from build123d import *

# Parameters (mm, degrees)
SKETCH1_R           = 2
BOSS_EXTRUDE1_DEPTH = 2.5
FILLET1_R           = 4
FILLET3_R           = 12


with BuildPart() as part:
    # Sketch1 → Boss-Extrude1 (new body)
    with BuildSketch(Plane(origin=(0, 0, 0), x_dir=(1, 0, 0), z_dir=(0, 1, 0))):
        Polygon((-14.798836476, 8.869056619), (-26.798836476, 8.869056619), (-26.798836476, -35.130943381), (199.665714924, -35.130943381), (199.665714924, 8.869056619), (187.665714924, 8.869056619), (187.665714924, -23.130943381), (-14.798836476, -23.130943381), align=None)
        with Locations(Location((-20.798836476, 2.869056619, 0), (0, 0, 270))):
            Circle(SKETCH1_R, mode=Mode.SUBTRACT)
        with Locations(Location((-20.798836476, -29.130943381, 0), (0, 0, 270))):
            Circle(SKETCH1_R, mode=Mode.SUBTRACT)
        with Locations(Location((193.665714924, 2.869056619, 0), (0, 0, 270))):
            Circle(SKETCH1_R, mode=Mode.SUBTRACT)
        with Locations(Location((193.665714924, -29.130943381, 0), (0, 0, 270))):
            Circle(SKETCH1_R, mode=Mode.SUBTRACT)
    extrude(amount=BOSS_EXTRUDE1_DEPTH)

    # Fillet1
    fillet1_edges = [part.edges().sort_by_distance(p)[0] for p in [
        (-26.798836476, 1.25, -8.869056619),
        (-14.798836476, 1.25, -8.869056619),
        (187.665714924, 1.25, -8.869056619),
        (199.665714924, 1.25, -8.869056619),
        (199.665714924, 1.25, 35.130943381),
        (-26.798836476, 1.25, 35.130943381),
    ]]
    fillet(fillet1_edges, radius=FILLET1_R)

    # Fillet3
    fillet3_edges = [part.edges().sort_by_distance(p)[0] for p in [
        (-14.798836476, 1.25, 23.130943381),
        (187.665714924, 1.25, 23.130943381),
    ]]
    fillet(fillet3_edges, radius=FILLET3_R)


solid = part.part
Verification items for the finished model (mm, model axes). A direction names the side the tool comes from. Coordinates: 2 decimals unless noted, no trailing zeros. Order: outer loops, then holes, each group sorted by start corner. A loop starts at its lowest first (then second) coordinate and runs counter-clockwise, first axis right, second up. Notation, with made-up numbers: (62.25, -6.5) -> (106.25, -6.5) arc R22 ccw to (106.25, 21.5) -> close; hole circle Ø5 at (56, 77.5). An arc over 180 degrees is marked (long way). Put each result on its own line as item: value. Start each with the question number.
1. Cross-section at A-A, the plane z = 3.5. Record the boundary of the cut face in (x, y).
2. Mould release check, pull along X, two halves, no side actions. Record for faces 1 (the cylindrical face through (-25.596, 1.268, -7.728)), 2 (the cylindrical face through (-11.4, 1.3, 19.5)), 3 (the flat face through (86, 2.5, 24)): released by +X, released by -X, zero draft, split by the parting line, or undercut.
3. Go/stop test with a flat-tipped pin: pin 1 Ø1 at (x, y) = (44.5, 1.5) entering from -Z. Record where the tip stops, or that it passes through.
4. Cross-section at D-D, the plane x = 15.5. Record the boundary of the cut face in (y, z).
5. Access from +Z, -Z, +X, -X, +Y, -Y to the whole of each face (thin tool, end or side, straight path). Record for faces 4 (the cylindrical face through (-22.75, 1.23, -3.3)), 5 (the cylindrical face through (-16.002, 1.268, -7.728)).
6. Material ranges on L1, parallel to X at y = 0.6, z = -3.5; L2, parallel to X at y = 2.45, z = 0; L3, parallel to X at y = 0.95, z = 30, recorded low to high. Write a range as [from, to].
7. Cross-section at C-C, the plane z = 14.5. Record the boundary of the cut face in (x, y).
8. Cross-section at B-B, the plane y = 2.05. Record the boundary of the cut face in (x, z), then the cut area to 3 significant figures.
Computed:
1. outline: (-26.8, 0) -> (-14.8, 0) -> (-14.8, 2.5) -> (-26.8, 2.5) -> close; (187.67, 0) -> (199.67, 0) -> (199.67, 2.5) -> (187.67, 2.5) -> close
2. face 1: released by -X
2. face 2: undercut
2. face 3: zero draft
3. pin 1: z = 23.13
4. outline: (0, 23.13) -> (2.5, 23.13) -> (2.5, 35.13) -> (0, 35.13) -> close
5. face 4: +Y, -Y
5. face 5: -Z, +Y, -Y
6. L1: [-26.8, -22.7], [-18.9, -14.8], [187.67, 191.77], [195.56, 199.67]
6. L2: [-26.8, -14.8], [187.67, 199.67]
6. L3: [-26.8, -22.6], [-19, 191.86], [195.47, 199.67]
7. outline: (-26.8, 0) -> (-14.32, 0) -> (-14.32, 2.5) -> (-26.8, 2.5) -> close; (187.18, 0) -> (199.67, 0) -> (199.67, 2.5) -> (187.18, 2.5) -> close
8. outline: (-26.8, -4.87) arc R4 ccw to (-22.8, -8.87) -> (-18.8, -8.87) arc R4 ccw to (-14.8, -4.87) -> (-14.8, 11.13) arc R12 cw to (-2.8, 23.13) -> (175.67, 23.13) arc R12 cw to (187.67, 11.13) -> (187.67, -4.87) arc R4 ccw to (191.67, -8.87) -> (195.67, -8.87) arc R4 ccw to (199.67, -4.87) -> (199.67, 31.13) arc R4 ccw to (195.67, 35.13) -> (-22.8, 35.13) arc R4 ccw to (-26.8, 31.13) -> close; hole circle Ø4 at (-20.8, -2.87); hole circle Ø4 at (-20.8, 29.13); hole circle Ø4 at (193.67, -2.87); hole circle Ø4 at (193.67, 29.13)
8. area: 3,480 mm2
